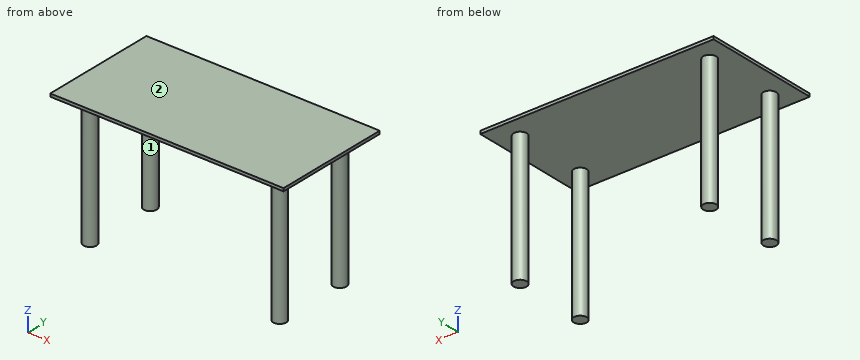
```python
from build123d import *

# Parameters (mm, degrees)
F0_W     = 1600
F0_H     = 800
F1_DEPTH = 20
F2_R     = 45
F3_DEPTH = 900
F4_ANGLE = 180


with BuildPart() as f1:
    # F0 (on Top) → F1 (new body)
    with BuildSketch(Plane.XY):
        Rectangle(F0_W, F0_H)
    extrude(amount=F1_DEPTH)

    # F2 (on face) → F3 (join)
    with BuildSketch(Plane.XY.offset(20)):
        with Locations((-650, 250)):
            Circle(F2_R)
        with Locations((650, 250)):
            Circle(F2_R)
        with Locations((-650, -250)):
            Circle(F2_R)
        with Locations((650, -250)):
            Circle(F2_R)
    extrude(amount=F3_DEPTH)


with BuildPart() as f1_1:
    # F4: moved
    add(f1.part.rotate(Axis((0, -400, 20), (1, 0, 0)), F4_ANGLE))


solid = f1_1.part
```
Source: CAD feature listing. Evaluate the final solid. Frame: model axes, mm. Face numbers are marked on the shaded views. Give positions to 0.01 mm unless a question says otherwise; leave off trailing zeros. Order: outer loops, then holes, each group sorted by start corner. A loop starts at its lowest first (then second) coordinate and runs counter-clockwise, first axis right, second up. Notation, with made-up numbers: (44, 47.5) -> (60, 47.5) arc R32 ccw to (60, 75.5) -> close; hole circle Ø9 at (77.25, -30.75). An arc over 180 degrees is marked (long way). Use a Markdown table: item, result.
Q1. Section A-A (x = -650). Return the cut outline in (y, z), and give its area (3 significant figures).
A:
| item | result |
|---|---|
| outline | (-1200, 20) -> (-1095, 20) -> (-1095, -880) -> (-1005, -880) -> (-1005, 20) -> (-595, 20) -> (-595, -880) -> (-505, -880) -> (-505, 20) -> (-400, 20) -> (-400, 40) -> (-1200, 40) -> close |
| area | 178,000 mm^2 |
Q2. First-contact query: P1, Ø1.5, axis at x = 612, z = -539.5, coming from the +Y side; P2, Ø12, axis at x = 120, y = -908.5, coming from the -Z side. Flat tips, straight axial feed; report the tip coordinate or a pass-through.
A:
| item | result |
|---|---|
| P1 | y = -524.75 |
| P2 | z = 20 |
Q3. Material intervals for line 1 (Z direction, x = 38.5, y = -838.5); line 2 (Y direction, x = -647.5, z = -512); line 3 (X direction, y = -1028.5, z = -843), sorted ascending. Write a range as [from, to].
A:
| item | result |
|---|---|
| line 1 | [20, 40] |
| line 2 | [-1094.93, -1005.07], [-594.93, -505.07] |
| line 3 | [-689.53, -610.47], [610.47, 689.53] |
Q4. Pull-direction query (X, two-part tool) for the marked faces 1 and 2; classes: +X half, -X half, draft (parallel to the pull), parting line (faces both ways), or undercut.
A:
| item | result |
|---|---|
| face 1 | undercut |
| face 2 | draft |
Q5. Section B-B (y = -1050). Return the cut outline in (x, z).
A:
| item | result |
|---|---|
| outline | (-800, 20) -> (-695, 20) -> (-695, -880) -> (-605, -880) -> (-605, 20) -> (605, 20) -> (605, -880) -> (695, -880) -> (695, 20) -> (800, 20) -> (800, 40) -> (-800, 40) -> close |
Q6. Section D-D (x = -57.5). Return the cut outline in (y, z), and give its area (3 significant figures).
A:
| item | result |
|---|---|
| outline | (-1200, 20) -> (-400, 20) -> (-400, 40) -> (-1200, 40) -> close |
| area | 16,000 mm^2 |
Q7. Section C-C (z = -264). Return the cut outline in (x, y), and give its area (3 significant figures).
A:
| item | result |
|---|---|
| outline | circle Ø90 at (-650, -1050); circle Ø90 at (-650, -550); circle Ø90 at (650, -1050); circle Ø90 at (650, -550) |
| area | 25,400 mm^2 |
